Verification items for the finished model (mm, model axes). A direction names the side the tool comes from. Coordinates: 2 decimals unless noted, no trailing zeros. Order: outer loops, then holes, each group sorted by start corner. A loop starts at its lowest first (then second) coordinate and runs counter-clockwise, first axis right, second up. Notation, with made-up numbers: (33, 57.25) -> (73, 57.25) arc R13 ccw to (73, 69.25) -> close; hole circle Ø3 at (38, -13). An arc over 180 degrees is marked (long way). Answer as CSV lines item,"result".
```python
from build123d import *

# Parameters (mm, degrees)
SKETCH_W            = 30
SKETCH_H            = 15
PAD_DEPTH           = 3.5
SKETCH001_W         = 30
SKETCH001_H         = 15
SKETCH001_W_2       = 25
SKETCH001_H_2       = 12.5
PAD001_DEPTH        = 7.5
POCKET_DEPTH        = 15.001
LINEARPATTERN_COUNT = 2
LINEARPATTERN_PITCH = 15
SKETCH003_W         = 8
SKETCH003_H         = 7.5
POCKET001_DEPTH     = 1.25
SKETCH004_W         = 4.5
SKETCH004_H         = 12.5
PAD002_DEPTH        = 3.5
SKETCH005_R         = 1.5
PAD003_DEPTH        = 2
SKETCH006_W         = 28
SKETCH006_H         = 13
POCKET002_DEPTH     = 2
SKETCH007_W         = 0.5
SKETCH007_H         = 5
PAD004_DEPTH        = 1
CHAMFER_SIZE        = 0.49


with BuildPart() as part:
    # Sketch → Pad (new body)
    with BuildSketch(Plane.XY):
        Rectangle(SKETCH_W, SKETCH_H)
    extrude(amount=PAD_DEPTH)

    # Sketch001 → Pad001 (new body)
    with BuildSketch(Plane.XY.offset(3.5)):
        Rectangle(SKETCH001_W, SKETCH001_H)
        Rectangle(SKETCH001_W_2, SKETCH001_H_2, mode=Mode.SUBTRACT)
    extrude(amount=PAD001_DEPTH)

    # Sketch002 → Pocket (cut, through all)
    with BuildSketch(Plane.XZ.offset(7.5)):
        with BuildLine():
            Line((-9, 0.722949), (-9, 0))
            Line((-9, 0), (-6, 0))
            Line((-6, 0), (-6, 0.722949))
            ThreePointArc((-6, 0.722949), (-5.37226, 1.668412), (-5.285841, 2.8))
            Line((-9.714159, 2.8), (-5.285841, 2.8))
            ThreePointArc((-9.714159, 2.8), (-9.62774, 1.668412), (-9, 0.722949))
        make_face()
    pocket = extrude(amount=-POCKET_DEPTH, mode=Mode.SUBTRACT)

    # LinearPattern: Pocket ×2
    with Locations(*[(i * LINEARPATTERN_PITCH, 0, 0) for i in range(1, LINEARPATTERN_COUNT)]):
        add(pocket, mode=Mode.SUBTRACT)

    # Sketch003 → Pocket001 (cut)
    with BuildSketch(Plane.XZ.offset(7.5)):
        with Locations((0, 7.25)):
            Rectangle(SKETCH003_W, SKETCH003_H)
    extrude(amount=-POCKET001_DEPTH, mode=Mode.SUBTRACT)

    # Sketch004 → Pad002 (new body)
    with BuildSketch(Plane.XY.offset(3.5)):
        with Locations((-10.25, 0)):
            Rectangle(SKETCH004_W, SKETCH004_H)
        with Locations((10.25, 0)):
            Rectangle(SKETCH004_W, SKETCH004_H)
    extrude(amount=PAD002_DEPTH)

    # Sketch005 → Pad003 (new body)
    with BuildSketch(Plane.XY.offset(7)):
        with Locations((-10, 0)):
            Circle(SKETCH005_R)
        with Locations((10, 0)):
            Circle(SKETCH005_R)
    extrude(amount=PAD003_DEPTH)

    # Sketch006 → Pocket002 (cut)
    with BuildSketch(Plane.XY.offset(11)):
        Rectangle(SKETCH006_W, SKETCH006_H)
    extrude(amount=-POCKET002_DEPTH, mode=Mode.SUBTRACT)

    # Sketch007 → Pad004 (new body)
    with BuildSketch(Plane.XY.offset(11)):
        with Locations((-13.75, 0)):
            Rectangle(SKETCH007_W, SKETCH007_H)
        with Locations((13.75, 0)):
            Rectangle(SKETCH007_W, SKETCH007_H)
    extrude(amount=-PAD004_DEPTH)

    # Chamfer
    chamfer_edges = [part.edges().sort_by_distance(p)[0] for p in [
        (-13.5, 0, 11),
        (13.5, 0, 11),
    ]]
    chamfer(chamfer_edges, length=CHAMFER_SIZE)


solid = part.part
```
Item 1: Tool access check on faces 4 (the cylindrical face through (-5.38, -0.11, 1.65)), 5 (the flat face through (14, -0.1, 9.8)), 6 (the flat face through (4, -7, 7)), 7 (the flat face through (-8, 0, 5)), 8 (the flat face through (-1, 7, 11)). Record the directions out of +Z, -Z, +X, -X, +Y, -Y that give a thin tool (end or side, any length) a straight path to the whole face; none if there is none.
Answer list:
face 4,"+Y, -Y"
face 5,"none"
face 6,"+Z, -Y"
face 7,"+Z"
face 8,"+Z, +X, -X, +Y, -Y"
Item 2: Release check for a two-part mould opening along Z. For faces 1 (the flat face through (12, 0, 0)), 2 (the flat face through (15, 0, 5)), 3 (the cylindrical face through (9.62, -0.11, 1.65)) record: +Z half, -Z half, draft (parallel to the pull), parting line (faces both ways), or undercut.
Answer list:
face 1,"-Z half"
face 2,"draft"
face 3,"undercut"
Item 3: Section check B-B, the plane x = -0.5. Record the boundary of the cut face in (y, z).
Answer list:
outline,"(-7.5, 0) -> (7.5, 0) -> (7.5, 11) -> (6.5, 11) -> (6.5, 9) -> (6.25, 9) -> (6.25, 3.5) -> (-7.5, 3.5) -> close"
Item 4: Thickness scan on line 1 (X direction, y = 5.5, z = 2.25) (3 decimals); line 2 (Y direction, x = -5, z = 4.25); line 3 (X direction, y = 2.75, z = 4.25). Record the ranges inside material, lowest first.
Answer list:
line 1,"-15 to -9.745, -5.255 to 5.255, 9.745 to 15"
line 2,"-7.5 to -6.25, 6.25 to 7.5"
line 3,"-15 to -8, 8 to 15"
Item 5: Depth check by flat-ended pin: pin 1 Ø3 at (x, z) = (2, 6) entering from -Y; pin 2 Ø1.3 at (x, y) = (-9, 3) entering from +Z; pin 3 Ø2.5 at (x, y) = (-10, 0) entering from +Z. Enter the tip coordinate at first touch or a pass-through.
Answer list:
pin 1,"y = 6.25"
pin 2,"z = 7"
pin 3,"z = 9"
Item 6: Section check A-A, the plane z = 6.5. Record the boundary of the cut face in (x, y), plus the area to 3 significant figures.
Answer list:
outline,"(-15, -7.5) -> (-4, -7.5) -> (-4, -6.25) -> (-8, -6.25) -> (-8, 6.25) -> (8, 6.25) -> (8, -6.25) -> (4, -6.25) -> (4, -7.5) -> (15, -7.5) -> (15, 7.5) -> (-15, 7.5) -> close"
area,"240 mm2"
